Geometry: see drawing. Coordinates: mm, zero at the bounding-box minimum. A direction names the side the tool comes from. Give positions to 0.01 mm unless a question says otherwise; leave off trailing zeros. One line per question, with ' | ' between items.
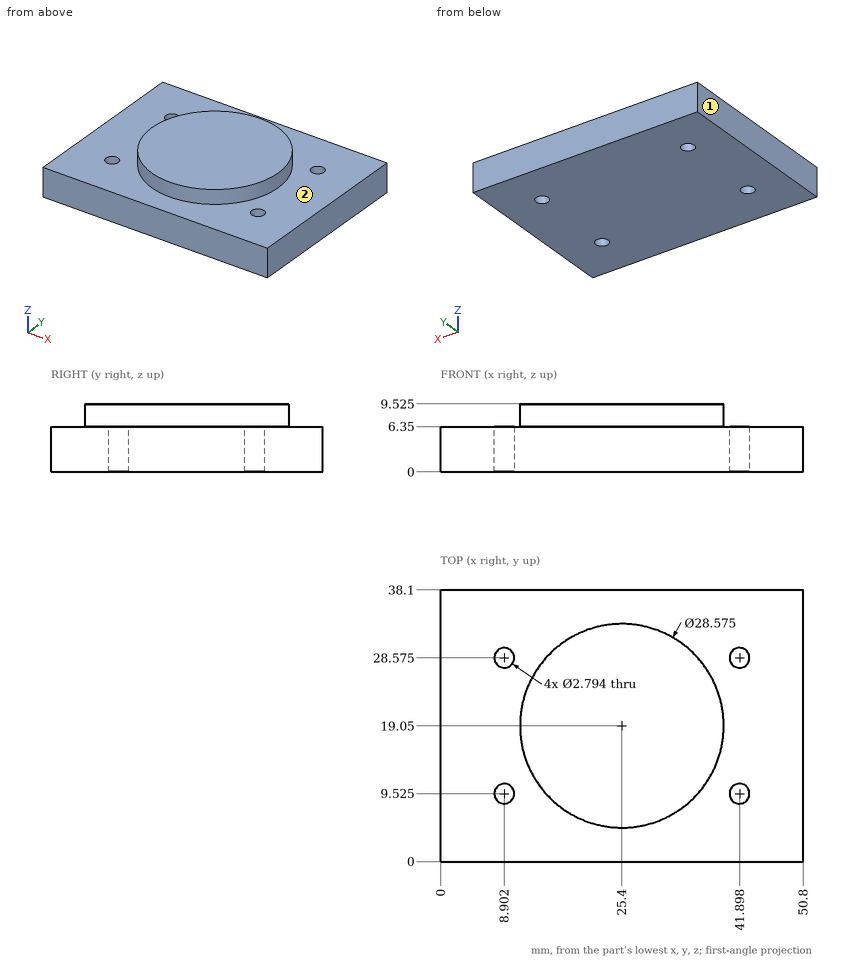
1. Pin query (flat end, axial travel): P1, Ø3.5, axis at x = 41.9, y = 28.58, coming from the +Z side; P2, Ø1, axis at y = 6, z = 6, coming from the -X side. Return the tip coordinate at first contact, or that it passes through.
Determined:
P1: stops at z = 6.35 | P2: stops at x = 0
2. Ray query, line 1 along X through (y, z) = (28.5, 2.75); line 2 along Y through (x, z) = (42, 1.25); line 3 along Y through (x, z) = (42.5, 2.5) (1 decimal). Return the intervals inside material, ascending. Write a range as from..to.
Determined:
line 1: x = 0..7.51, 10.3..40.5, 43.29..50.8 | line 2: y = 0..8.13, 10.92..27.18, 29.97..38.1 | line 3: y = 0..8.3, 10.8..27.3, 29.8..38.1
3. Reachability of the marked faces 1 and 2 from +Z, -Z, +X, -X, +Y, -Y: full face, straight path, thin tool, end or side. Return the list, or none.
Determined:
face 1: +Z, -Z, -X, +Y, -Y | face 2: +Z
